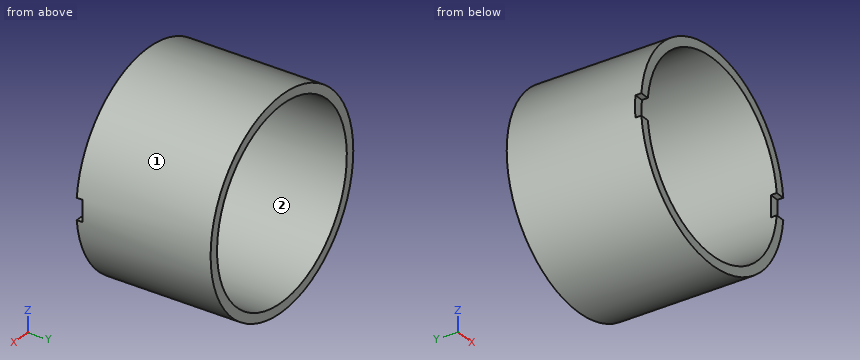
```python
from build123d import *

# Parameters (mm, degrees)
BOSS_EXTRUDE1_DEPTH      = 12.97
BOSS_EXTRUDE1_DEPTH_BACK = 0.6
SKETCH1_R                = 10.5
SKETCH1_R_2              = 9.55
CUT_EXTRUDE1_DEPTH       = 20.716006188
CUT_EXTRUDE1_DEPTH_BACK  = 20.716006188
SKETCH2_W                = 2.16
SKETCH2_H                = 0.617422303


with BuildPart() as part:
    # Sketch1 → Boss-Extrude1 (new, two sides: drawn at the far end of the back side and taken through both)
    with BuildSketch(Plane(origin=(0, 0, 0), x_dir=(1, 0, 0), z_dir=(0, 1, 0)).offset(-BOSS_EXTRUDE1_DEPTH_BACK)):
        with Locations(Location((0, 0, 0), (0, 0, 270))):
            Circle(SKETCH1_R)
        with Locations(Location((0, 0, 0), (0, 0, 270))):
            Circle(SKETCH1_R_2, mode=Mode.SUBTRACT)
    extrude(amount=BOSS_EXTRUDE1_DEPTH + BOSS_EXTRUDE1_DEPTH_BACK)

    # Sketch2 → Cut-Extrude1 (cut, two sides: drawn at the far end of the back side and taken through both)
    with BuildSketch(Plane(origin=(0, 0, 0), x_dir=(0, 0, -1), z_dir=(1, 0, 0)).offset(-CUT_EXTRUDE1_DEPTH_BACK)):
        with Locations((0, -0.308711152)):
            Rectangle(SKETCH2_W, SKETCH2_H)
    extrude(amount=CUT_EXTRUDE1_DEPTH + CUT_EXTRUDE1_DEPTH_BACK, mode=Mode.SUBTRACT)


solid = part.part
```
Source: CAD feature listing. Evaluate the final solid. Frame: model axes, mm. Face numbers are marked on the shaded views. Coordinates: 2 decimals unless noted, no trailing zeros. Loops run counter-clockwise (first coordinate to the right, second up) from the corner with the lowest first, then second, coordinate; pieces in that order, holes last. Notation, with made-up numbers: (9.25, 77.25) - (37.25, 77.25) arc R27 cw to (37.25, 106.25) - close; hole circle Ø8 at (26, -27). An arc over 180 degrees is marked (long way). Answer as CSV lines item,"result".
1. Section A-A (z = 0). Return loops of the section in (x, y).
Established:
outline,"(-10.5, 0) - (-9.55, 0) - (-9.55, 12.97) - (-10.5, 12.97) - close; (9.55, 0) - (10.5, 0) - (10.5, 12.97) - (9.55, 12.97) - close"
2. Section C-C (y = 5). Return loops of the section in (x, z), then the cut area to 3 significant figures.
Established:
outline,"circle Ø21 at (0, 0); hole circle Ø19.1 at (0, 0)"
area,"59.8 mm2"
3. Mould query, pull axis X, two halves, no side actions, for the marked faces 1 and 2. Classes: released by +X, released by -X, zero draft, split by the parting line, or undercut.
Established:
face 1,"split by the parting line"
face 2,"undercut"
4. Contact query for flat-ended pins moving along their axis: pin 1 (0.8 mm diameter, centred on x = -10, z = 0.5, fed in from -Y); pin 2 (2 mm diameter, centred on y = 6, z = 1.5, fed in from +X); pin 3 (1 mm diameter, centred on y = 7, z = -4, fed in from -X). Output: stop coordinate, or through.
Established:
pin 1,"stops at y = 0"
pin 2,"stops at x = 10.49"
pin 3,"stops at x = -9.9"
5. Section B-B (x = 0). Return loops of the section in (y, z).
Established:
outline,"(-0.6, -10.5) - (12.97, -10.5) - (12.97, -9.55) - (-0.6, -9.55) - close; (-0.6, 9.55) - (12.97, 9.55) - (12.97, 10.5) - (-0.6, 10.5) - close"
6. Ray query, line 1 (X direction, y = 4.5, z = 0); line 2 (X direction, y = 6, z = -3.75); line 3 (Z direction, x = 5.25, y = 7). Return the intervals inside material, ascending.
Established:
line 1,"x = -10.5 to -9.55, 9.55 to 10.5"
line 2,"x = -9.81 to -8.78, 8.78 to 9.81"
line 3,"z = -9.09 to -7.98, 7.98 to 9.09"
